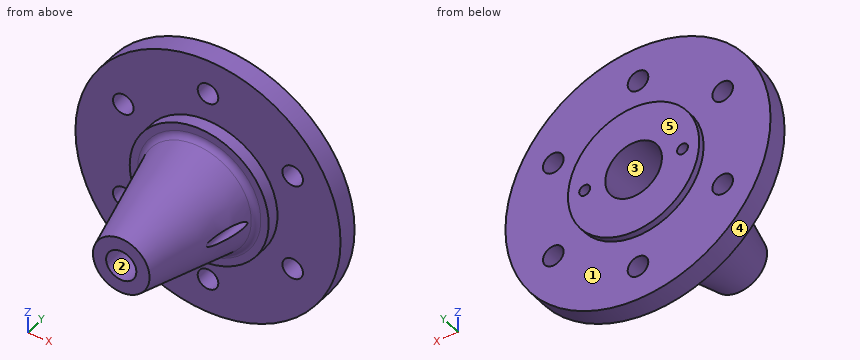
from build123d import *

# Parameters (mm, degrees)
FILLET1_R                 = 5
F_1_0_16_DIAMETER_HOLE1_D = 16
CIRPATTERN1_COUNT         = 6
M10X1_5_TAPPED_HOLE1_D    = 8.5


# Read off the part's stored shape, not the designer's step: Cut-Revolve-Thin1
with BuildPart() as part:
    # Sketch1 → Revolve1 (revolve)
    with BuildSketch(Plane.XY, mode=Mode.PRIVATE) as revolve1_sk:
        Polygon((0, 0), (51, 0), (51, -5), (103, -5), (103, -21), (54, -21), (54, -31), (44, -31), (22, -120), (0, -120), align=None)
    revolve(revolve1_sk.sketch.rotate(Axis((0, 0, 0), (0, -1, 0)), 180), axis=Axis((0, 0, 0), (0, -1, 0)))

    # Cut-Revolve-Thin1 outline → Cut-Revolve-Thin1 (revolve, cut)
    with BuildSketch(Plane.XY):
        Polygon((0, -120), (11.75, -120), (11.75, -82), (16, -79.240017729), (16, -65.247037966), (11, -62), (11, -51.143483525), (22, -44), (22, 0), (0, 0), align=None)
    revolve(axis=Axis((0, 0, 0), (0, 1, 0)), mode=Mode.SUBTRACT)

    # Fillet1
    fillet1_edges = [part.edges().sort_by_distance(p)[0] for p in [
        (44, -31, 0),
    ]]
    fillet(fillet1_edges, radius=FILLET1_R)

    # Ø1.0 (16) Diameter Hole1 (through all)
    with Locations(Plane(origin=(0, -5, 0), x_dir=(1, 0, 0), z_dir=(0, 1, 0))):
        with Locations((0, 76)):
            f_1_0_16_diameter_hole1 = Hole(F_1_0_16_DIAMETER_HOLE1_D / 2)

    # CirPattern1: Ø1.0 (16) Diameter Hole1 ×6 about axis
    cirpattern1_axis = Axis((0, 0, 0), (0, 1, 0))
    for i in range(1, CIRPATTERN1_COUNT):
        add(f_1_0_16_diameter_hole1.rotate(cirpattern1_axis, i * 360 / CIRPATTERN1_COUNT), mode=Mode.SUBTRACT)

    # M10x1.5 Tapped Hole1 (through all)
    with Locations(Plane(origin=(0, 0, 0), x_dir=(1, 0, 0), z_dir=(0, 1, 0))):
        with Locations((38, 0), (-38, 0)):
            Hole(M10X1_5_TAPPED_HOLE1_D / 2)


solid = part.part
Check sheet for the modelled part. Datum: model origin and axes. Units: mm. Face numbers are marked on the shaded views. A direction names the side the tool comes from. Coordinates: 2 decimals unless noted, no trailing zeros. Write each loop counter-clockwise with the first axis right and the second up, starting at its lowest first coordinate (ties: lowest second). Pieces come first, ordered by that corner, then holes.
Item 1: Cross-section at D-D on x = -87. Record the boundary of the cut face in (y, z), then the cut area to 3 significant figures.
Numbers:
outline: (-21, -55.14) - (-5, -55.14) - (-5, 55.14) - (-21, 55.14) - close
area: 1,760 mm2
Item 2: Access from +Z, -Z, +X, -X, +Y, -Y to the whole of each face (thin tool, end or side, straight path). Record for the marked faces 1 and 2.
Numbers:
face 1: +Y
face 2: -Y
Item 3: Cross-section at C-C on y = -94.5. Record the boundary of the cut face in (x, z), then the cut area to 3 significant figures.
Numbers:
outline: circle Ø56.61 at (0, 0); hole circle Ø23.5 at (0, 0)
area: 2,080 mm2
Item 4: Scan lines: probe 1 along Y at (x, z) = (-85, 33.5); probe 2 along X at (y, z) = (-20, -32.5); probe 3 along X at (y, z) = (-85, 9). Record each from-to range of solid material in increasing order.
Numbers:
probe 1: y = -21 to -5
probe 2: x = -97.74 to -71.63, -60.01 to 60.01, 71.63 to 97.74
probe 3: x = -29.3 to -7.55, 7.55 to 29.3
Item 5: Cross-section at A-A on z = 76. Record the boundary of the cut face in (x, y), then the cut area to 3 significant figures.
Numbers:
outline: (-69.52, -21) - (-8, -21) - (-8, -5) - (-69.52, -5) - close; (8, -21) - (69.52, -21) - (69.52, -5) - (8, -5) - close
area: 1,970 mm2
Item 6: Mould release check, pull along Z, two halves, no side actions. Record for the marked faces 3, 4 and 5: released by +Z, released by -Z, zero draft, split by the parting line, or undercut.
Numbers:
face 3: undercut
face 4: split by the parting line
face 5: zero draft
Item 7: Depth check by flat-ended pin: pin 1 Ø18.5 at (x, z) = (0, 76) entering from +Y; pin 2 Ø21 at (x, z) = (65.82, -38) entering from -Y; pin 3 Ø3 at (x, y) = (-11.5, -74) entering from +Z. Enter the tip coordinate at first touch or a pass-through.
Numbers:
pin 1: stops at y = -5
pin 2: stops at y = -21
pin 3: stops at z = 31.98
Item 8: Cross-section at B-B on z = -38. Count the separate pieces of the cut face and the enclosed holes in it, then the cut area to 3 significant figures.
Numbers:
separate pieces: 3
enclosed holes: 0
area: 4,380 mm2
